Design review of the part built by this model. Coordinates are the model's own, in mm. A direction names the side the tool comes from. Coordinates: 2 decimals unless noted, no trailing zeros. Order: outer loops, then holes, each group sorted by start corner. A loop starts at its lowest first (then second) coordinate and runs counter-clockwise, first axis right, second up. Notation, with made-up numbers: (-5, 24.5) -> (7, 24.5) arc R21 cw to (7, 40.5) -> close; hole circle Ø2 at (78, 74.25). An arc over 180 degrees is marked (long way). Write item = value, one per line.
```python
from build123d import *

# Parameters (mm, degrees)
SKETCH1_R                      = 27.4955
SKETCH1_R_2                    = 52.3875
SKETCH1_R_3                    = 3.3
BOSS_EXTRUDE1_DEPTH            = 3.81
M8_CLEARANCE_HOLE1_D           = 9
M8_CLEARANCE_HOLE1_CSINK_D     = 9.05
M8_CLEARANCE_HOLE1_CSINK_ANGLE = 90
CIRPATTERN1_COUNT              = 9
CUT_EXTRUDE2_DEPTH             = 705.3211269
CIRPATTERN3_COUNT              = 11
CIRPATTERN3_ANGLE              = 320


with BuildPart() as part:
    # Sketch1 → Boss-Extrude1 (new, symmetric)
    with BuildSketch(Plane(origin=(0, 0, 0), x_dir=(-1, 0, 0), z_dir=(0, 1, 0))):
        with BuildLine():
            Line((-663.344331246, 5.11591187), (-571.334153098, 11.036768117))
            ThreePointArc((-571.334153098, 11.036768117), (-571.018141837, 11.05791522), (-570.70224289, 11.080678619))
            Line((-570.70224289, 11.080678619), (-458.651128563, 19.443128234))
            ThreePointArc((-458.651128563, 19.443128234), (-453.955105952, 21.098716352), (-450.736142738, 24.897647282))
            Line((-450.736142738, 24.897647282), (-396.525446728, 140.500644454))
            ThreePointArc((-396.525446728, 140.500644454), (-393.715871596, 171.819021526), (-411.692336104, 197.617881552))
            ThreePointArc((-411.692336104, 197.617881552), (-413.372500119, 198.071242365), (-414.950136715, 197.336701751))
            Line((-414.950136715, 197.336701751), (-420.215020333, 192.071818133))
            ThreePointArc((-420.215020333, 192.071818133), (-427.298656721, 190.662795249), (-431.31121441, 196.668012211))
            Line((-431.31121441, 196.668012211), (-431.31121441, 203.240745001))
            ThreePointArc((-431.31121441, 203.240745001), (-431.968379704, 204.945600851), (-433.59982344, 205.768273949))
            ThreePointArc((-433.59982344, 205.768273949), (-438.15, 205.994), (-442.70017656, 205.768273949))
            ThreePointArc((-442.70017656, 205.768273949), (-444.331620296, 204.945600851), (-444.98878559, 203.240745001))
            Line((-444.98878559, 203.240745001), (-444.98878559, 196.668012211))
            ThreePointArc((-444.98878559, 196.668012211), (-451.48878559, 190.168012211), (-457.98878559, 196.668012211))
            Line((-457.98878559, 196.668012211), (-457.98878559, 197.245022653))
            ThreePointArc((-457.98878559, 197.245022653), (-459.278285753, 199.455870942), (-461.837486501, 199.421924563))
            ThreePointArc((-461.837486501, 199.421924563), (-464.019895008, 198.024699819), (-466.120112298, 196.506730383))
            Line((-466.120112298, 196.506730383), (-526.629683433, 150.121113421))
            ThreePointArc((-526.629683433, 150.121113421), (-551.530592574, 139.247052869), (-578.312485484, 134.661130809))
            ThreePointArc((-578.312485484, 134.661130809), (-592.081443241, 132.419097692), (-604.99890828, 127.151270133))
            ThreePointArc((-604.99890828, 127.151270133), (-612.407574664, 124.492595217), (-620.274454537, 124.229743629))
            Line((-620.274454537, 124.229743629), (-661.161974504, 129.250099814))
            ThreePointArc((-661.161974504, 129.250099814), (-670.249252048, 125.077827159), (-670.600960367, 115.084690838))
            Line((-670.600960367, 115.084690838), (-649.054093444, 77.225755025))
            ThreePointArc((-649.054093444, 77.225755025), (-647.394780527, 71.225067939), (-648.786811147, 65.156804956))
            Line((-648.786811147, 65.156804956), (-672.43464209, 18.961557425))
            ThreePointArc((-672.43464209, 18.961557425), (-671.918273078, 9.393648822), (-663.344331246, 5.11591187))
        make_face()
        with Locations(Location((-438.15, 160.02, 0), (0, 0, 270))):
            Circle(SKETCH1_R, mode=Mode.SUBTRACT)
        with Locations(Location((-575.31, 72.821477372, 0), (0, 0, 270))):
            Circle(SKETCH1_R_2, mode=Mode.SUBTRACT)
        with Locations(Location((-662.32278, 119.79609772, 0), (0, 0, 270))):
            Circle(SKETCH1_R_3, mode=Mode.SUBTRACT)
        with Locations(Location((-663.956, 14.621251755, 0), (0, 0, 270))):
            Circle(SKETCH1_R_3, mode=Mode.SUBTRACT)
        with Locations(Location((-459.360014272, 28.941712658, 0), (0, 0, 270))):
            Circle(SKETCH1_R_3, mode=Mode.SUBTRACT)
    extrude(amount=BOSS_EXTRUDE1_DEPTH, both=True)

    # M8 Clearance Hole1 (through all)
    with Locations(Plane(origin=(0, -3.81, 0), x_dir=(-1, 0, 0), z_dir=(0, -1, 0))):
        with Locations((-438.15, -199.019999978)):
            m8_clearance_hole1 = CounterSinkHole(M8_CLEARANCE_HOLE1_D / 2, M8_CLEARANCE_HOLE1_CSINK_D / 2, counter_sink_angle=M8_CLEARANCE_HOLE1_CSINK_ANGLE)

    # CirPattern1: M8 Clearance Hole1 ×9 about axis
    cirpattern1_axis = Axis((438.15, 0, 160.02), (0, 1, 0))
    for i in range(1, CIRPATTERN1_COUNT):
        add(m8_clearance_hole1.rotate(cirpattern1_axis, i * 360 / CIRPATTERN1_COUNT), mode=Mode.SUBTRACT)

    # Sketch10 → Cut-Extrude2 (cut, through all)
    with BuildSketch(Plane.XZ.offset(3.81)):
        with BuildLine():
            Line((460.055399035, 108.47079033), (501.653528527, 82.025066826))
            ThreePointArc((501.653528527, 82.025066826), (507.74174649, 75.794215969), (510.419523322, 67.504498748))
            ThreePointArc((510.419523322, 67.504498748), (511.336032734, 60.722893264), (512.959284307, 54.07494495))
            ThreePointArc((512.959284307, 54.07494495), (509.569281047, 36.661622947), (493.298252827, 29.592708892))
            Line((493.298252827, 29.592708892), (477.784713934, 30.750494677))
            ThreePointArc((477.784713934, 30.750494677), (473.468249432, 32.15763422), (470.293491627, 35.40306491))
            ThreePointArc((470.293491627, 35.40306491), (466.5665587, 39.399041065), (461.505556985, 41.459166331))
            ThreePointArc((461.505556985, 41.459166331), (457.342507431, 43.270498962), (454.490842485, 46.803191211))
            Line((454.490842485, 46.803191211), (436.590721722, 84.974765498))
            ThreePointArc((436.590721722, 84.974765498), (435.154253671, 96.778102142), (440.996916533, 107.134041843))
            ThreePointArc((440.996916533, 107.134041843), (444.966962938, 109.594428804), (449.557948705, 110.453278114))
            Line((449.557948705, 110.453278114), (453.24181467, 110.453278114))
            ThreePointArc((453.24181467, 110.453278114), (456.789884205, 109.947588368), (460.055399035, 108.47079033))
        make_face()
        with BuildLine():
            Line((488.447021855, 135.568616467), (518.5458141, 116.433517192))
            ThreePointArc((518.5458141, 116.433517192), (523.526027217, 115.31070897), (528.083819046, 117.610655627))
            ThreePointArc((528.083819046, 117.610655627), (531.194244853, 120.677331811), (534.503353276, 123.528481221))
            ThreePointArc((534.503353276, 123.528481221), (536.820485804, 129.284400418), (533.124064721, 134.267991506))
            ThreePointArc((533.124064721, 134.267991506), (526.661398117, 137.399578344), (520.391516426, 140.901217866))
            Line((520.391516426, 140.901217866), (497.676544793, 158.314132116))
            ThreePointArc((497.676544793, 158.314132116), (491.351665893, 159.127989595), (487.50938857, 154.038455032))
            ThreePointArc((487.50938857, 154.038455032), (486.663269024, 149.130057447), (485.330309415, 144.330942547))
            ThreePointArc((485.330309415, 144.330942547), (485.381225421, 139.4135911), (488.447021855, 135.568616467))
        make_face()
        with BuildLine():
            Line((635.420385908, 116.492899074), (643.506881083, 117.485795833))
            ThreePointArc((643.506881083, 117.485795833), (652.594158627, 113.313523178), (652.945866946, 103.320386857))
            Line((652.945866946, 103.320386857), (647.859361663, 94.383139612))
            ThreePointArc((647.859361663, 94.383139612), (641.819407992, 91.195500663), (636.38230144, 95.328290853))
            ThreePointArc((636.38230144, 95.328290853), (633.867295103, 101.236717058), (630.78232235, 106.868564021))
            ThreePointArc((630.78232235, 106.868564021), (630.473854175, 112.946950119), (635.420385908, 116.492899074))
        make_face()
        with BuildLine():
            Line((644.438689484, 15.877190959), (626.45783883, 17.03425895))
            ThreePointArc((626.45783883, 17.03425895), (620.947612088, 21.069043166), (622.282896399, 27.766736666))
            ThreePointArc((622.282896399, 27.766736666), (629.718866036, 37.099523997), (635.326028557, 47.633008334))
            ThreePointArc((635.326028557, 47.633008334), (640.940766472, 51.521041328), (646.833678916, 48.069133834))
            Line((646.833678916, 48.069133834), (655.044052135, 32.030444107))
            ThreePointArc((655.044052135, 32.030444107), (654.441621622, 20.86788407), (644.438689484, 15.877190959))
        make_face()
    extrude(amount=-CUT_EXTRUDE2_DEPTH, mode=Mode.SUBTRACT)

    # Sketch14 → 5.0mm Dowel Hole2 (revolve, cut)
    with BuildSketch(Plane(origin=(575.31, 3.81, 129.971477372), x_dir=(0, 0, 1), z_dir=(1, 0, 0))):
        Polygon((0, 0), (0, 9.122151548), (2.5, 7.62), (2.5, 0), align=None)
    f_5_0mm_dowel_hole2 = revolve(axis=Axis((575.31, 10.16, 129.971477372), (0, -1, 0)), mode=Mode.SUBTRACT)

    # CirPattern3: 5.0mm Dowel Hole2 ×11 about axis
    cirpattern3_axis = Axis((575.31, 0, 72.821477372), (0, 1, 0))
    for i in range(1, CIRPATTERN3_COUNT):
        add(f_5_0mm_dowel_hole2.rotate(cirpattern3_axis, i * CIRPATTERN3_ANGLE / (CIRPATTERN3_COUNT - 1)), mode=Mode.SUBTRACT)


solid = part.part
```
(1) Insertion check: pin 1 (0.6 mm diameter, centred on y = -1, z = 197, fed in from -X); pin 2 (2 mm diameter, centred on y = -0.5, z = 200.5, fed in from -X). Each pin has a flat end and moves straight along its axis. Give the tip position at first contact, or say it passes through.
Report:
pin_1 = 410.43
pin_2 = 431.31
(2) For L1, parallel to X at y = -2.5, z = 36.5; L2, parallel to X at y = 1.5, z = 189; L3, parallel to X at y = -0.5, z = 60, list the stretches that pass through material, from the lowest coordinate up.
Report:
L1 = 445.3 to 469.57, 509.44 to 537.56, 613.06 to 618.12, 622.57 to 629.32, 652.76 to 663.46
L2 = 402.46 to 408.67, 417.49 to 458.81, 467.63 to 475.91
L3 = 434.28 to 448.3, 511.48 to 517.57, 522.15 to 524.52, 626.1 to 651.43
(3) The part is to be moulded in two halves that separate along X. For faces 1 (the cylindrical face through (393.6, 0.05, 171.38)), 2 (the cylindrical face through (551.165, 0.053, 139.357)), 3 (the cylindrical face through (640.84, -0.053, 51.516)), say which applies: released by +X, released by -X, zero draft, split by the parting line, or undercut.
Report:
face_1 = released by -X
face_2 = released by +X
face_3 = undercut
(4) For faces 4 (the cylindrical face through (457.394, -0.053, 43.232)), 5 (the flat face through (660.445, 0.053, 42.383)), 6 (the flat face through (444.989, 0, 200)), 7 (the flat face through (496, 0.1, 173.6)), list the 3-axis set-ups (+Z, -Z, +X, -X, +Y, -Y) from which the entire face can be reached by the end or side of a thin tool; tool diameter is ignored.
Report:
face_4 = +Y, -Y
face_5 = +X, +Y, -Y
face_6 = +Z, +Y, -Y
face_7 = +Z, +X, +Y, -Y
(5) We need section A-A (z = 177). Write out the cut boundary in (x, y), and give its area (3 significant figures).
Report:
outline = (395.43, -3.81) -> (416.52, -3.81) -> (416.52, 3.81) -> (395.43, 3.81) -> close; (459.78, -3.81) -> (491.57, -3.81) -> (491.57, 3.81) -> (459.78, 3.81) -> close
area = 403 mm²
(6) We need section B-B (y = 0.5). Give the number of separate pieces and of enclosed holes in the cut face, and give its area (3 significant figures).
Report:
separate_pieces = 1
enclosed_holes = 29
area = 16,400 mm²
